Geometry check sheet. Reference: the model listing, model coordinates, mm. Coordinates: 2 decimals unless noted, no trailing zeros. Write each loop counter-clockwise with the first axis right and the second up, starting at its lowest first coordinate (ties: lowest second). Pieces come first, ordered by that corner, then holes.
from build123d import *

# Parameters (mm, degrees)
F1_DEPTH = 6.35
F3_D     = 6.7564


with BuildPart() as f1:
    # F0 (on Top) → F1 (new body)
    with BuildSketch(Plane.XY):
        Polygon((38.1, 76.2), (-31.8138207153, 76.2), (-38.1, 69.9138207153), (-38.1, -76.2), (38.1, -76.2), align=None)
    extrude(amount=F1_DEPTH)

    # F3 (through all)
    with Locations(Plane.XY.offset(6.35)):
        with Locations((-25.4, 63.5)):
            Hole(F3_D / 2)


solid = f1.part
1. Sectioned sample at A-A, the plane x = -25.4. Record the boundary of the cut face in (y, z).
Computed values:
outline: (-76.2, 0) - (60.12, 0) - (60.12, 6.35) - (-76.2, 6.35) - close; (66.88, 0) - (76.2, 0) - (76.2, 6.35) - (66.88, 6.35) - close
2. Thickness scan on line 1 along Y through (x, z) = (-25.4, 4.5). Record the ranges inside material, lowest first.
Computed values:
line 1: y = -76.2 to 60.12, 66.88 to 76.2
3. Draft check along X on faces 1 (the flat face through (-1, 1, 6.35)), 2 (the flat face through (-34.913, 73.101, 3.131)), 3 (the cylindrical face through (-24.67, 60.2, 3.13)). Enter one of: released by +X, released by -X, zero draft, split by the parting line, or undercut.
Computed values:
face 1: zero draft
face 2: released by -X
face 3: undercut
4. Sectioned sample at B-B, the plane y = 63.5. Record the boundary of the cut face in (x, z).
Computed values:
outline: (-38.1, 0) - (-28.78, 0) - (-28.78, 6.35) - (-38.1, 6.35) - close; (-22.02, 0) - (38.1, 0) - (38.1, 6.35) - (-22.02, 6.35) - close
